from build123d import *

# Parameters (mm, degrees)
SKETCH1_W           = 15
SKETCH1_H           = 16
BOSS_EXTRUDE1_DEPTH = 5
SKETCH2_R           = 4.15
CUT_EXTRUDE1_DEPTH  = 2
SKETCH4_W           = 4
SKETCH4_H           = 4
CUT_EXTRUDE2_DEPTH  = 4
SKETCH8_W           = 13
SKETCH8_H           = 1.5
CUT_EXTRUDE4_DEPTH  = 10
SKETCH9_R           = 9
CUT_EXTRUDE6_DEPTH  = 50
FILLET2_R           = 1
FILLET3_R           = 1


with BuildPart() as part:
    # Sketch1 → Boss-Extrude1 (new body)
    with BuildSketch(Plane.XY):
        Rectangle(SKETCH1_W, SKETCH1_H)
    extrude(amount=BOSS_EXTRUDE1_DEPTH)

    # Sketch2 → Cut-Extrude1 (cut)
    with BuildSketch(Plane.XY.offset(5)):
        Circle(SKETCH2_R)
    extrude(amount=-CUT_EXTRUDE1_DEPTH, mode=Mode.SUBTRACT)

    # Sketch4 → Cut-Extrude2 (cut)
    with BuildSketch(Plane(origin=(7.5, 0, 0), x_dir=(0, 0, -1), z_dir=(1, 0, 0))):
        with Locations((-5, 0)):
            Rectangle(SKETCH4_W, SKETCH4_H)
    extrude(amount=-CUT_EXTRUDE2_DEPTH, mode=Mode.SUBTRACT)

    # Sketch8 → Cut-Extrude4 (cut)
    with BuildSketch(Plane.XY.offset(5)):
        with Locations((0, 5.75)):
            Rectangle(SKETCH8_W, SKETCH8_H)
        with Locations((0, -5.75)):
            Rectangle(SKETCH8_W, SKETCH8_H)
    extrude(amount=-CUT_EXTRUDE4_DEPTH, mode=Mode.SUBTRACT)

    # Sketch9 → Cut-Extrude6 (cut)
    with BuildSketch(Plane.ZY.offset(7.5)):
        with Locations((-7, 0)):
            Circle(SKETCH9_R)
    extrude(amount=-CUT_EXTRUDE6_DEPTH, mode=Mode.SUBTRACT)

    # Fillet2
    fillet2_edges = [part.edges().sort_by_distance(p)[0] for p in [
        (0, 8, 5),
    ]]
    fillet(fillet2_edges, radius=FILLET2_R)

    # Fillet3
    fillet3_edges = [part.edges().sort_by_distance(p)[0] for p in [
        (0, -8, 5),
    ]]
    fillet(fillet3_edges, radius=FILLET3_R)


solid = part.part
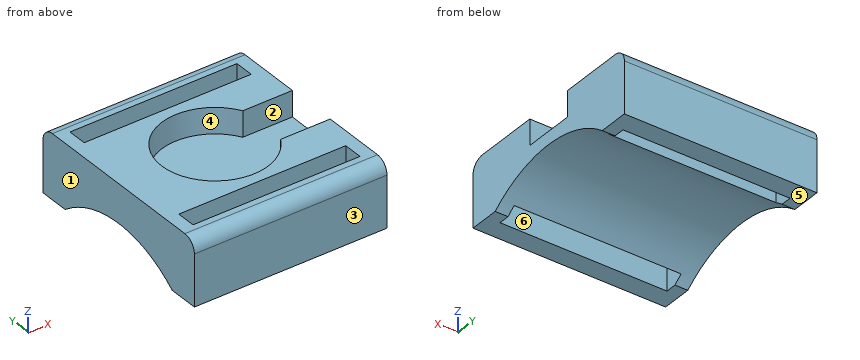
For this review, take the finished solid that the model builds, in its own axes (mm). Face numbers are marked on the shaded views. A direction names the side the tool comes from. Give positions to 0.01 mm unless a question says otherwise; leave off trailing zeros. Order: outer loops, then holes, each group sorted by start corner. A loop starts at its lowest first (then second) coordinate and runs counter-clockwise, first axis right, second up. Notation, with made-up numbers: (-25, -29.5) - (-2, -29.5) arc R18 ccw to (-2, -14.5) - close; hole circle Ø1 at (6.5, 74.5). An arc over 180 degrees is marked (long way). Answer as a JSON object with one key per item and string values. Group by question number.
Item 1: Take a section at B-B on z = 0.7. Give the boundary of the cut face in (x, y), and give its area (3 significant figures).
Item 2: Take a section at D-D on z = 3.2. Give the boundary of the cut face in (x, y), and give its area (3 significant figures).
Item 3: Machinability: for the marked faces 4, 5 and 6, which of the approach directions +Z, -Z, +X, -X, +Y, -Y give a long, thin tool a straight path to every point of the face, cutting with its end or side? Answer none if there is none.
Item 4: Wall thickness on line 1 along Y through (x, z) = (-6, 3.5); line 2 along Y through (x, z) = (0, 3.8); line 3 along Y through (x, z) = (6.25, 3.7): over which ranges is each line inside the solid? List them lowest first.
Item 5: Take a section at A-A on y = 6. Give the boundary of the cut face in (x, z), and give its area (3 significant figures).
Item 6: Take a section at C-C on x = 0. Give the boundary of the cut face in (y, z).
Item 7: Draft analysis for pull direction Y (two halves, no side actions). For the marked faces 1, 2 and 3, state which applies: pulls with the +Y half, pulls with the -Y half, needs draft (parallel to the pull), parting line crosses it, or undercut.
Item 8: Clearance check with flat-ended pins moving along their axes: pin 1 Ø6.5 at (x, y) = (0, 0) entering from -Z; pin 2 Ø0.6 at (x, z) = (6, 4.5) entering from -Y; pin 3 Ø8 at (x, y) = (6, -0.5) entering from -Z. State where each tip first meets the part, or that it passes through.
Reported:
{
 "1": {"outline": "(-7.5, -8) - (7.5, -8) - (7.5, -4.66) - (-7.5, -4.66) - close; (-7.5, 4.66) - (7.5, 4.66) - (7.5, 8) - (-7.5, 8) - close; hole (-6.5, -6.5) - (6.5, -6.5) - (6.5, -5) - (-6.5, -5) - close; hole (-6.5, 5) - (6.5, 5) - (6.5, 6.5) - (-6.5, 6.5) - close", "area": "61.2 mm^2"},
 "2": {"outline": "(-7.5, -8) - (7.5, -8) - (7.5, -2) - (3.64, -2) arc R4.15 cw (long way) to (3.64, 2) - (7.5, 2) - (7.5, 8) - (-7.5, 8) - close; hole (-6.5, -6.5) - (6.5, -6.5) - (6.5, -5) - (-6.5, -5) - close; hole (-6.5, 5) - (6.5, 5) - (6.5, 6.5) - (-6.5, 6.5) - close", "area": "133 mm^2"},
 "3": {"face 4": "+Z", "face 5": "-Z, +X, -X, +Y, -Y", "face 6": "+Z, -Z"},
 "4": {"line 1": "-8 to -6.5, -5 to 5, 6.5 to 8", "line 2": "-8 to -6.5, -5 to -4.15, 4.15 to 5, 6.5 to 8", "line 3": "-8 to -6.5, -5 to -2, 2 to 5, 6.5 to 8"},
 "5": {"outline": "(-7.5, 0) - (-6.5, 0) - (-6.5, 5) - (-7.5, 5) - close; (6.5, 0) - (7.5, 0) - (7.5, 5) - (6.5, 5) - close", "area": "10.0 mm^2"},
 "6": {"outline": "(-8, 0) - (-6.5, 0) - (-6.5, 5) - (-7, 5) arc R1 ccw to (-8, 4) - close; (-5, 0.48) arc R9 cw to (5, 0.48) - (5, 5) - (4.15, 5) - (4.15, 3) - (-4.15, 3) - (-4.15, 5) - (-5, 5) - close; (6.5, 0) - (8, 0) - (8, 4) arc R1 ccw to (7, 5) - (6.5, 5) - close"},
 "7": {"face 1": "needs draft", "face 2": "undercut", "face 3": "pulls with the -Y half"},
 "8": {"pin 1": "z = 1.39", "pin 2": "y = -7.98", "pin 3": "z = 0.79"}
}
